Could you check a few things on this model? Use its own coordinates, in mm. Round coordinates to 2 decimals unless told otherwise and drop trailing zeros. Loops run counter-clockwise (first coordinate to the right, second up) from the corner with the lowest first, then second, coordinate; pieces in that order, holes last. Notation, with made-up numbers: (57.5, 24.5) -> (75.5, 24.5) arc R13 cw to (75.5, 35.5) -> close; hole circle Ø3 at (-0.5, 72). An arc over 180 degrees is marked (long way). One line per item, written item: value.
Autodesk Inventor part; units mm, degrees
ref_plane "YZ Plane" through (0, 0, 0) normal (1, 0, 0) x (0, 1, 0)
ref_plane "XZ Plane" through (0, 0, 0) normal (0, 1, 0) x (-1, 0, 0)
ref_plane "XY Plane" through (0, 0, 0) normal (0, 0, 1) x (1, 0, 0)
sketch "Sketch1" plane through (0, 0, 0) normal (0, 0, 1) x (1, 0, 0)
  line L0 (266.7, 89.6306) -> (523.875, 89.6306)
  line L1 (523.875, 89.6306) -> (523.875, 26.1306)
  line L2 (523.875, 26.1306) -> (266.7, 26.1306)
  line L3 (266.7, 89.6306) -> (266.7, 76.9306)
  line L4 (266.7, 76.9306) -> (247.65, 76.9306)
  line L5 (247.65, 76.9306) -> (247.65, 64.2306)
  line L6 (247.65, 64.2306) -> (266.7, 64.2306)
  line L7 (266.7, 64.2306) -> (266.7, 51.5306)
  line L8 (266.7, 51.5306) -> (247.65, 51.5306)
  line L9 (247.65, 51.5306) -> (247.65, 38.8306)
  line L10 (247.65, 38.8306) -> (266.7, 38.8306)
  line L11 (266.7, 38.8306) -> (266.7, 26.1306)
  point P0 (0, 0)
  dimension "d4" = 63.5
  dimension "d17" = 257.175
  dimension "d18" = 19.05
  dimension "d19" = 12.7
  dimension "d20" = 12.7
  dimension "d21" = 12.7
  dimension "d22" = 12.7
  dimension "d23" = 12.7
  dimension "d24" = 0
extrude "Extrusion1" add sketch "Sketch1" along normal blind 19.05
mirror "Mirror1" about plane through (523.875, 26.1306, 0) normal (1, 0, 0) of "Extrusion1"
sketch "Sketch3" plane through (0, 0, 19.05) normal (0, 0, 1) x (1, 0, 0)
  line L0 (266.7, 89.6306) -> (781.05, 89.6306)
  line L1 (781.05, 89.6306) -> (781.05, 80.1056)
  line L2 (781.05, 80.1056) -> (266.7, 80.1056)
  line L3 (266.7, 80.1056) -> (266.7, 89.6306)
  point P0 (0, 0)
  dimension "d25" = 9.525
extrude "Extrusion3" cut sketch "Sketch3" against normal blind 9.525
properties part number "top_cover_side" material "Wood (Birch)"
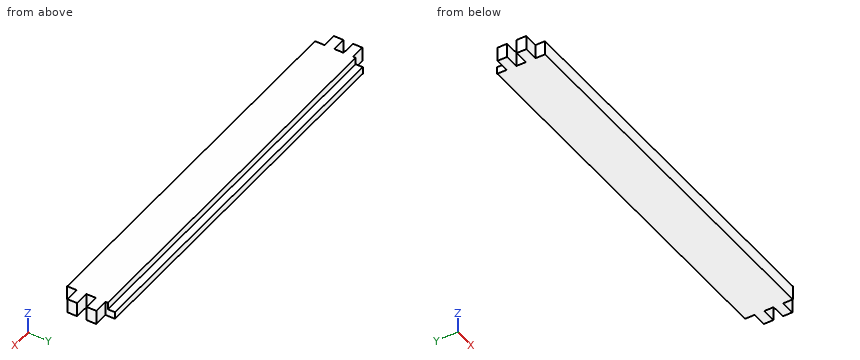
(1) If we section it at A-A, the plane x = 420: Please give me the cut outline in (y, z) (3 decimals).
Recorded:
outline: (26.131, 0) -> (89.631, 0) -> (89.631, 9.525) -> (80.106, 9.525) -> (80.106, 19.05) -> (26.131, 19.05) -> close
(2) If I drill on L1, parallel to Y at x = 300, z = 10.75; L2, parallel to X at y = 29, z = 1; L3, parallel to Z at x = 305.5, y = 81 (3 decimals), over which ranges is the centre line in solid material (lowest first)?
Recorded:
L1: 26.13 to 80.11
L2: 266.7 to 781.05
L3: 0 to 9.525
(3) If we section it at B-B, the plane z = 4: Please give me the cut outline in (x, y), then the cut area to 3 significant figures.
Recorded:
outline: (247.65, 38.83) -> (266.7, 38.83) -> (266.7, 26.13) -> (781.05, 26.13) -> (781.05, 38.83) -> (800.1, 38.83) -> (800.1, 51.53) -> (781.05, 51.53) -> (781.05, 64.23) -> (800.1, 64.23) -> (800.1, 76.93) -> (781.05, 76.93) -> (781.05, 89.63) -> (266.7, 89.63) -> (266.7, 76.93) -> (247.65, 76.93) -> (247.65, 64.23) -> (266.7, 64.23) -> (266.7, 51.53) -> (247.65, 51.53) -> close
area: 33,600 mm²
(4) If we section it at C-C, the plane y = 58: Please give me the cut outline in (x, z), then the cut area to 3 significant figures.
Recorded:
outline: (266.7, 0) -> (781.05, 0) -> (781.05, 19.05) -> (266.7, 19.05) -> close
area: 9,800 mm²
(5) I'm going to push flat-ended pins straight in: pin 1 Ø5 at (x, y) = (636, 84.5) entering from +Z (3 decimals); pin 2 Ø5.5 at (x, z) = (253.5, 6.5) entering from -Y; pin 3 Ø6.5 at (y, z) = (59.5, 5) entering from -X. Where does each tip first touch, or does it pass through?
Recorded:
pin 1: z = 9.525
pin 2: y = 38.83
pin 3: x = 266.7
